```python
from build123d import *

# Parameters (mm, degrees)
F0_R     = 11.125
F1_DEPTH = 7


with BuildPart() as f1:
    # F0 (on Front) → F1 (new body)
    with BuildSketch(Plane.XZ):
        with BuildLine():
            ThreePointArc((-11.425942, 27.229862), (-12.149095, 20.2237), (-17.614547, 15.780944))
            ThreePointArc((-17.614547, 15.780944), (-33.50268, 8.942403), (-33.395492, -8.354617))
            ThreePointArc((-33.395492, -8.354617), (-18.787986, -14.339204), (-7.403348, -3.403733))
            ThreePointArc((-7.403348, -3.403733), (0.487123, -2.044763), (8.377595, -3.403733))
            ThreePointArc((8.377595, -3.403733), (18.572382, -14.304901), (32.513153, -8.973477))
            ThreePointArc((32.513153, -8.973477), (32.772871, 9.130893), (15.494492, 14.543222))
            ThreePointArc((15.494492, 14.543222), (11.160472, 20.161243), (10.543607, 27.229862))
            ThreePointArc((10.543607, 27.229862), (13.432728, 43.194843), (0, 52.293714))
            ThreePointArc((0, 52.293714), (-12.910225, 43.042824), (-11.425942, 27.229862))
        make_face()
        with Locations((-21.5418, 0)):
            Circle(F0_R, mode=Mode.SUBTRACT)
        with Locations((21.5418, 0)):
            Circle(F0_R, mode=Mode.SUBTRACT)
        with Locations((0, 12.686641)):
            Circle(F0_R, mode=Mode.SUBTRACT)
        with Locations((0, 37.686641)):
            Circle(F0_R, mode=Mode.SUBTRACT)
    extrude(amount=F1_DEPTH)


solid = f1.part
```
Read the model definition and answer for the solid it produces. Units are mm, in the model's axes. Coordinates: 2 decimals unless noted, no trailing zeros. Write each loop counter-clockwise with the first axis right and the second up, starting at its lowest first coordinate (ties: lowest second). Pieces come first, ordered by that corner, then holes. Notation, with made-up numbers: (-14, 15) -> (33, 15) arc R30 cw to (33, 54) -> close; hole circle Ø10 at (23, 67). An arc over 180 degrees is marked (long way). Write item = value, one per line.
(1) For a pull along Z with two mould halves and no side action, classify faces 1 (the face through (18.357, -3.451, -14.253)), 2 (the face through (-2.412, -3.451, 26.826)), 3 (the face through (32.93, -3.45, 8.91)) as +Z half, -Z half, draft (parallel to the pull), parting line (faces both ways), or undercut.
From the geometry:
face_1 = -Z half
face_2 = undercut
face_3 = parting line
(2) Section D-D on x = 13.5 is taken. Write down the section's boundary in (y, z).
From the geometry:
outline = (-7, -11.93) -> (0, -11.93) -> (0, -7.69) -> (-7, -7.69) -> close; (-7, 7.69) -> (0, 7.69) -> (0, 16.35) -> (-7, 16.35) -> close; (-7, 31.83) -> (0, 31.83) -> (0, 43.03) -> (-7, 43.03) -> close
(3) Section A-A on z = 0 is taken. Write down the section's boundary in (x, y), plus the area to 3 significant figures.
From the geometry:
outline = (-36.05, -7) -> (-32.67, -7) -> (-32.67, 0) -> (-36.05, 0) -> close; (-10.42, -7) -> (10.42, -7) -> (10.42, 0) -> (-10.42, 0) -> close; (32.67, -7) -> (35.65, -7) -> (35.65, 0) -> (32.67, 0) -> close
area = 190 mm2
(4) Section B-B on y = -4.75 is taken. Count the separate pieces of the cut face and the enclosed holes in it, plus the area to 3 significant figures.
From the geometry:
separate_pieces = 1
enclosed_holes = 4
area = 1,030 mm2
(5) Straight lines are drawn through the part: L1, parallel to X at y = -5.75, z = -3.5; L2, parallel to Z at x = -8.5, y = -2.25; L3, parallel to X at y = -3, z = -7. For each, find the intervals that lie inside material, in ascending order. Write a range as from..to.
From the geometry:
L1 = -35.57..-32.1, -10.98..-7.43, 8.39..10.98, 32.1..35.18
L2 = -6.49..5.51, 19.86..30.51, 44.86..48.77
L3 = -34.21..-30.19, -12.9..-8.76, 9.49..12.9, 30.19..33.8
(6) Given pin 1 Ø1 at (y, z) = (-6, 33) entering from +X; pin 2 Ø1 at (y, z) = (-3, 44) entering from +X; pin 3 Ø18 at (x, z) = (21.54, 0) entering from +Y; pin 4 Ø3 at (x, y) = (-20, -4.5) entering from -Z, each flat-ended and moving along its own axis, determine where each tip first touches the part or whether it passes through.
From the geometry:
pin_1 = 14.07
pin_2 = 13.3
pin_3 = through
pin_4 = -14.59
(7) Section C-C on x = 24 is taken. Write down the section's boundary in (y, z).
From the geometry:
outline = (-7, -14.43) -> (0, -14.43) -> (0, -10.85) -> (-7, -10.85) -> close; (-7, 10.85) -> (0, 10.85) -> (0, 14.99) -> (-7, 14.99) -> close
